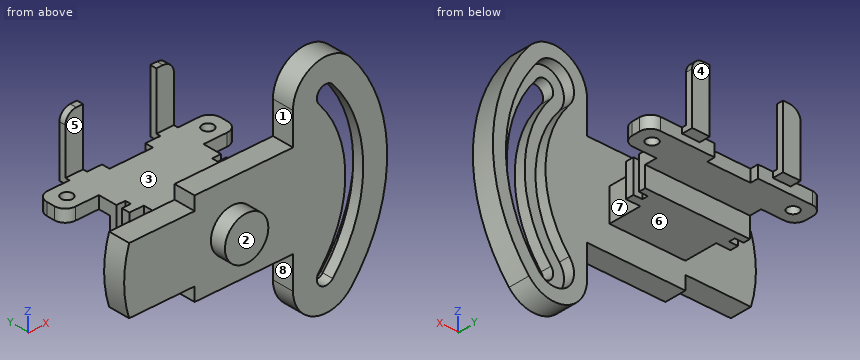
from build123d import *

# Parameters (mm, degrees)
BOSS_EXTRUDE1_DEPTH    = 1.125
M1_8_CLEARANCE_HOLE1_D = 2.1
BOSS_EXTRUDE3_DEPTH    = 4
SKETCH10_R             = 4
BOSS_EXTRUDE4_DEPTH    = 2.8
CUT_EXTRUDE1_DEPTH     = 2
BOSS_EXTRUDE9_DEPTH    = 6
SKETCH21_W             = 3.25
SKETCH21_H             = 1
BOSS_EXTRUDE10_DEPTH   = 2
BOSS_EXTRUDE13_DEPTH   = 1.2
SKETCH25_W             = 14
SKETCH25_H             = 3.75
BOSS_EXTRUDE12_DEPTH   = 10


with BuildPart() as part:
    # Sketch1 → Boss-Extrude1 (new, symmetric)
    with BuildSketch(Plane.XY):
        with BuildLine():
            Line((-7, -8.85), (-7, -15))
            Line((-7, -15), (7, -15))
            Line((7, -15), (7, -8.85))
            Line((7, -8.85), (9.65, -8.85))
            Line((9.65, -8.85), (9.65, -7.35))
            Line((9.65, -7.35), (8, -7.35))
            Line((8, -7.35), (8, -6.25))
            Line((8, -6.25), (9.65, -6.25))
            Line((9.65, -6.25), (9.65, -2.75))
            Line((9.65, -2.75), (14, -2.75))
            ThreePointArc((14, -2.75), (15.414213562, -2.164213562), (16, -0.75))
            Line((16, -0.75), (16, 0.75))
            ThreePointArc((16, 0.75), (15.414213562, 2.164213562), (14, 2.75))
            Line((14, 2.75), (4, 2.75))
            Line((4, 2.75), (4, 1.25))
            Line((4, 1.25), (-4, 1.25))
            Line((-4, 1.25), (-4, 2.75))
            Line((-4, 2.75), (-14, 2.75))
            ThreePointArc((-14, 2.75), (-15.414213562, 2.164213562), (-16, 0.75))
            Line((-16, 0.75), (-16, -0.75))
            ThreePointArc((-16, -0.75), (-15.414213562, -2.164213562), (-14, -2.75))
            Line((-14, -2.75), (-9.65, -2.75))
            Line((-9.65, -2.75), (-9.65, -6.25))
            Line((-9.65, -6.25), (-8, -6.25))
            Line((-8, -6.25), (-8, -7.35))
            Line((-8, -7.35), (-9.65, -7.35))
            Line((-9.65, -7.35), (-9.65, -8.85))
            Line((-9.65, -8.85), (-7, -8.85))
        make_face()
    extrude(amount=BOSS_EXTRUDE1_DEPTH, both=True)

    # M1.8 Clearance Hole1 (through all)
    with Locations(Plane.XY.offset(1.125)):
        with Locations((-13, 0), (13, 0)):
            Hole(M1_8_CLEARANCE_HOLE1_D / 2)

    # Sketch8 → Boss-Extrude3 (add)
    with BuildSketch(Plane.XZ.offset(15)):
        with BuildLine():
            Line((-7, -7.125), (-7, -9.625))
            Line((-7, -9.625), (11.129010548, -9.625))
            Line((11.129010548, -9.625), (11.129010548, -15.548780253))
            ThreePointArc((11.129010548, -15.548780253), (15.116751021, -21.24386386), (21.832266629, -19.444446876))
            ThreePointArc((21.832266629, -19.444446876), (28.5, -1.125), (21.832266629, 17.194446876))
            ThreePointArc((21.832266629, 17.194446876), (15.116751021, 18.99386386), (11.129010548, 13.298780253))
            Line((11.129010548, 13.298780253), (11.129010548, 7.375))
            Line((11.129010548, 7.375), (-7, 7.375))
            Line((-7, 7.375), (-7, 4.875))
            Line((-7, 4.875), (-19.078784028, 4.875))
            ThreePointArc((-19.078784028, 4.875), (-20, -1.125), (-19.078784028, -7.125))
            Line((-19.078784028, -7.125), (-7, -7.125))
        make_face()
        with BuildLine():
            ThreePointArc((15.925618604, -14.488180697), (20.789418613, -1.125), (15.925618604, 12.238180697))
            ThreePointArc((15.925618604, 12.238180697), (16.128992379, 14.562753584), (18.453565266, 14.359379809))
            ThreePointArc((18.453565266, 14.359379809), (24.089418613, -1.125000171), (18.453565046, -16.609380071))
            ThreePointArc((18.453565046, -16.609380071), (16.128992248, -16.812753474), (15.925618604, -14.488180697))
        make_face(mode=Mode.SUBTRACT)
    extrude(amount=BOSS_EXTRUDE3_DEPTH)

    # Sketch10 → Boss-Extrude4 (add)
    with BuildSketch(Plane(origin=(0, -19, 0), x_dir=(-1, 0, 0), z_dir=(0, -1, 0))):
        with Locations(Location((0, 1.125, 0), (0, 0, 90))):
            Circle(SKETCH10_R)
    extrude(amount=BOSS_EXTRUDE4_DEPTH)

    # Sketch11 → Cut-Extrude1 (cut)
    with BuildSketch(Plane(origin=(0, -15, 0), x_dir=(1, 0, 0), z_dir=(0, 1, 0))):
        with BuildLine():
            ThreePointArc((14.393529718, -10.952605478), (18.789418613, 1.125), (14.393529718, 13.202605478))
            ThreePointArc((14.393529718, 13.202605478), (14.84341687, 18.344842227), (19.985653666, 17.894955608))
            ThreePointArc((19.985653666, 17.894955608), (26.089418613, 1.125000379), (19.985654153, -15.644955028))
            ThreePointArc((19.985654153, -15.644955028), (14.84341716, -16.09484247), (14.393529718, -10.952605478))
        make_face()
        with BuildLine():
            ThreePointArc((18.453565046, 16.609380071), (16.128992248, 16.812753474), (15.925618604, 14.488180697))
            ThreePointArc((15.925618604, 14.488180697), (20.789418613, 1.125), (15.925618604, -12.238180697))
            ThreePointArc((15.925618604, -12.238180697), (16.128992379, -14.562753584), (18.453565266, -14.359379809))
            ThreePointArc((18.453565266, -14.359379809), (24.089418613, 1.125000171), (18.453565046, 16.609380071))
        make_face(mode=Mode.SUBTRACT)
    extrude(amount=-CUT_EXTRUDE1_DEPTH, mode=Mode.SUBTRACT)

    # Sketch19 → Boss-Extrude9 (add)
    with BuildSketch(Plane.XY.offset(1.125)):
        Polygon((-9.65, -5), (-9.65, -6.25), (-8, -6.25), (-8, -7.35), (-9.65, -7.35), (-9.65, -8.85), (-6.6, -8.85), (-6.6, -5), align=None)
    boss_extrude9 = extrude(amount=-BOSS_EXTRUDE9_DEPTH)

    # Mirror1: Boss-Extrude9 across plane
    add(boss_extrude9.mirror(Plane(origin=(0, 0, 0), x_dir=(0, 0, 1), z_dir=(1, 0, 0))))

    # Sketch21 → Boss-Extrude10 (add)
    with BuildSketch(Plane(origin=(0, 2.75, 0), x_dir=(1, 0, 0), z_dir=(0, 1, 0))):
        with Locations((-8.375, -0.625)):
            Rectangle(SKETCH21_W, SKETCH21_H)
        with Locations((8.375, -0.625)):
            Rectangle(SKETCH21_W, SKETCH21_H)
    extrude(amount=BOSS_EXTRUDE10_DEPTH)

    # Sketch26 → Boss-Extrude13 (add)
    with BuildSketch(Plane(origin=(0, 4.75, 0), x_dir=(1, 0, 0), z_dir=(0, 1, 0))):
        with BuildLine():
            Line((-10, -0.125), (-6.75, -0.125))
            Line((-6.75, -0.125), (-6.75, -11.547583435))
            Line((-6.75, -11.547583435), (-8, -11.547583435))
            ThreePointArc((-8, -11.547583435), (-9.414213562, -10.961796997), (-10, -9.547583435))
            Line((-10, -9.547583435), (-10, -0.125))
        make_face()
        with BuildLine():
            Line((6.75, -0.125), (6.75, -11.547583435))
            Line((6.75, -11.547583435), (8, -11.547583435))
            ThreePointArc((8, -11.547583435), (9.414213562, -10.961796997), (10, -9.547583435))
            Line((10, -9.547583435), (10, -0.125))
            Line((10, -0.125), (6.75, -0.125))
        make_face()
    extrude(amount=-BOSS_EXTRUDE13_DEPTH)

    # Sketch25 → Boss-Extrude12 (add)
    with BuildSketch(Plane(origin=(0, -5, 0), x_dir=(1, 0, 0), z_dir=(0, 1, 0))):
        with Locations((0, 3)):
            Rectangle(SKETCH25_W, SKETCH25_H)
    extrude(amount=-BOSS_EXTRUDE12_DEPTH)


solid = part.part
Geometry: final body of the model. Coordinates: model frame, mm. Face numbers are marked on the shaded views. A direction names the side the tool comes from. Give positions to 0.01 mm unless a question says otherwise; leave off trailing zeros. Write each loop counter-clockwise with the first axis right and the second up, starting at its lowest first coordinate (ties: lowest second). Pieces come first, ordered by that corner, then holes. Notation, with made-up numbers: (83.5, 12) -> (122.5, 12) arc R32 ccw to (122.5, 49) -> close; hole circle Ø8 at (-15, -29.5). An arc over 180 degrees is marked (long way). Answer in a Markdown table with one row per item.
(1) Ray query, line 1 along Y through (x, z) = (-13, -0.6); line 2 along Y through (x, z) = (20, -19); line 3 along Z through (x, y) = (-14.5, -15.5) (3 decimals). Return the intervals inside material, ascending. Write a range as [from, to].
Answers below:
| item | result |
|---|---|
| line 1 | [-19, -15], [-2.75, -1.05], [1.05, 2.75] |
| line 2 | [-19, -15] |
| line 3 | [-7.125, 4.875] |
(2) Section query A-A on x = -13. Return loops of the section in (y, z) (3 decimals).
Answers below:
| item | result |
|---|---|
| outline | (-19, -7.125) -> (-15, -7.125) -> (-15, 4.875) -> (-19, 4.875) -> close; (-2.75, -1.125) -> (-1.05, -1.125) -> (-1.05, 1.125) -> (-2.75, 1.125) -> close; (1.05, -1.125) -> (2.75, -1.125) -> (2.75, 1.125) -> (1.05, 1.125) -> close |
(3) Draft query along Y for the marked faces 1, 2, 3 and 4. Return one class per face: +Y half, -Y half, draft (parallel to the pull), parting line (faces both ways), or undercut.
Answers below:
| item | result |
|---|---|
| face 1 | draft |
| face 2 | -Y half |
| face 3 | undercut |
| face 4 | +Y half |
(4) Section query C-C on z = 2. Return loops of the section in (x, y), then the cut area to 3 significant figures.
Answers below:
| item | result |
|---|---|
| outline | (-19.75, -19) -> (-2.5, -19) -> (-2.5, -21.8) -> (2.5, -21.8) -> (2.5, -19) -> (20.55, -19) -> (20.55, -17) -> (18.53, -17) -> (18.53, -15) -> (-19.75, -15) -> close; (-10, 3.55) -> (-6.75, 3.55) -> (-6.75, 4.75) -> (-10, 4.75) -> close; (6.75, 3.55) -> (10, 3.55) -> (10, 4.75) -> (6.75, 4.75) -> close; (23.89, -19) -> (28.33, -19) -> (28.33, -15) -> (25.9, -15) -> (25.9, -17) -> (23.89, -17) -> close |
| area | 193 mm^2 |
(5) Pin query (flat end, axial travel): pin 1 (1.8 mm diameter, centred on y = -11.5, z = -1, fed in from +X); pin 2 (10 mm diameter, centred on x = -12.5, z = 10, fed in from +Y); pin 3 (3 mm diameter, centred on x = -9, z = -1, fed in from -Y); pin 4 (2 mm diameter, centred on x = -15, y = -1, fed in from +Z) (3 decimals). Return the tip coordinate at first contact, or that it passes through.
Answers below:
| item | result |
|---|---|
| pin 1 | x = 7 |
| pin 2 | y = 4.75 |
| pin 3 | y = -19 |
| pin 4 | z = 1.125 |
(6) Section query D-D on x = 0. Return loops of the section in (y, z) (3 decimals).
Answers below:
| item | result |
|---|---|
| outline | (-21.8, -5.125) -> (-19, -5.125) -> (-19, -9.625) -> (-15, -9.625) -> (-15, -4.875) -> (-5, -4.875) -> (-5, -1.125) -> (1.25, -1.125) -> (1.25, 1.125) -> (-15, 1.125) -> (-15, 7.375) -> (-19, 7.375) -> (-19, 2.875) -> (-21.8, 2.875) -> close |
(7) Section query B-B on y = -17.75. Return loops of the section in (x, z) (3 decimals).
Answers below:
| item | result |
|---|---|
| outline | (-19.079, -7.125) -> (-7, -7.125) -> (-7, -9.625) -> (11.129, -9.625) -> (11.129, -15.549) arc R6.061 ccw to (21.832, -19.444) arc R28.5 ccw to (21.832, 17.194) arc R6.061 ccw to (11.129, 13.299) -> (11.129, 7.375) -> (-7, 7.375) -> (-7, 4.875) -> (-19.079, 4.875) arc R20 ccw to start; hole (15.926, -14.488) arc R1.65 ccw to (18.454, -16.609) arc R24.089 ccw to (18.454, 14.359) arc R1.65 ccw to (15.926, 12.238) arc R20.789 cw to start |
(8) Set-up query: the marked faces 5, 6, 7 and 8. Return all of +Z, -Z, +X, -X, +Y, -Y with unobstructed straight access to the full face (end or side cutting, diameter ignored); none if empty.
Answers below:
| item | result |
|---|---|
| face 5 | +Z, +X, -X |
| face 6 | -Z, +X, -X, +Y |
| face 7 | +Z, -Z, +X |
| face 8 | -Z, -X, +Y, -Y |
